Could you check a few things on this model? Use its own coordinates, in mm. Give positions to 0.01 mm unless a question says otherwise; leave off trailing zeros. Order: outer loops, then holes, each group sorted by start corner. A loop starts at its lowest first (then second) coordinate and runs counter-clockwise, first axis right, second up. Notation, with made-up numbers: (-39, 4) -> (0, 4) arc R8 cw to (0, 13) -> close; hole circle Ø8 at (23, 0). An arc over 180 degrees is marked (long way). Answer as CSV lines item,"result". Start each with the question number.
(1) I want a section at B-B (y = 171). Please give me the cut outline in (x, z).
(2) I need wall thicknesses on L1, parallel to X at y = 135, z = 15.75; L2, parallel to X at y = 187, z = 4; L3, parallel to Y at x = 120, z = 3.5. Which ranges of each line are inside material? Lowest first, please.
(3) I want a section at C-C (x = 147.5). Please give me the cut outline in (y, z).
(4) Will these pins go through, and if not, where does the flat tip stop? pin 1 Ø4 at (y, z) = (156, 5) entering from -X; pin 2 Ø2 at (y, z) = (214.5, 12.5) entering from -X; pin 3 Ø1.5 at (y, z) = (122.5, 14.5) entering from -X.
(5) I want a section at A-A (z = 9.5). Please give me the cut outline in (x, y), plus the area to 3 significant figures.
Autodesk Inventor part; units mm, degrees
ref_plane "YZ Plane" through (0, 0, 0) normal (1, 0, 0) x (0, 1, 0)
ref_plane "XZ Plane" through (0, 0, 0) normal (0, 1, 0) x (-1, 0, 0)
ref_plane "XY Plane" through (0, 0, 0) normal (0, 0, 1) x (1, 0, 0)
sketch "Sketch1" plane through (0, 0, 0) normal (0, 0, 1) x (1, 0, 0)
  line L0 (0, 0) -> (219, 0) construction
  line L1 (219, 0) -> (219, 18) construction
  line L2 (219, 18) -> (0, 18) construction
  line L3 (0, 18) -> (0, 0) construction
  line L4 (44.9362, 18) -> (174.0638, 18)
  line L5 (174.0638, 18) -> (174.0638, 40)
  line L6 (174.0638, 40) -> (44.9362, 40) construction
  line L7 (44.9362, 40) -> (44.9362, 18)
  line L8 (91.5484, 238) -> (127.4516, 238) construction
  arc A0 (123.9889, 226.8823) -> (95.0111, 226.8823) centre (109.5, 223) ccw
  line L9 (109.5, 238) -> (109.5, 292.3651) construction
  line L10 (44.9362, 40) -> (95.0111, 226.8823)
  line L11 (174.0638, 40) -> (123.9889, 226.8823)
  point P0 (109.5, 40)
  point P1 (109.5, 0)
  dimension "d2" = 18
  dimension "d3" = 219
  dimension "d4" = 40
  dimension "d5" = 220
  dimension "d6" = 15
  dimension "d7" = 75
extrude "Extrusion1" add sketch "Sketch1" along normal blind 18
properties part number "CPO-1-support"
Final values:
1,outline,"(80.04, 0) -> (138.96, 0) -> (138.96, 18) -> (80.04, 18) -> close"
2,L1,"70.39 to 148.61"
2,L2,"84.32 to 134.68"
2,L3,"18 to 233.71"
3,outline,"(18, 0) -> (139.14, 0) -> (139.14, 18) -> (18, 18) -> close"
4,pin 1,"x = 75.48"
4,pin 2,"x = 91.43"
4,pin 3,"x = 66.84"
5,outline,"(44.94, 18) -> (174.06, 18) -> (174.06, 40) -> (123.99, 226.88) arc R15 ccw to (95.01, 226.88) -> (44.94, 40) -> close"
5,area,"17,900 mm²"
